```python
from build123d import *

# Parameters (mm, degrees)
SKETCH1_R           = 1.7
SKETCH1_W           = 5.3
SKETCH1_H           = 7.2
BOSS_EXTRUDE2_DEPTH = 6
SKETCH1_4_W         = 5.3
SKETCH1_4_H         = 7.2
CUT_EXTRUDE1_DEPTH  = 3.8
FILLET2_R           = 4
FILLET3_R           = 2


with BuildPart() as part:
    # Sketch1 → Boss-Extrude2 (new body)
    # profile 1 of 2: a face of its own
    with BuildSketch(Plane(origin=(0, 0, 0), x_dir=(1, 0, 0), z_dir=(0, 1, 0))):
        Polygon((-25.7, 5), (-25.7, -5), (25.7, -5), (25.7, 5), (2.65, 5), (2.65, -2.2), (-2.65, -2.2), (-2.65, 5), align=None)
        with Locations(Location((-20, 0, 0), (0, 0, 270))):
            Circle(SKETCH1_R, mode=Mode.SUBTRACT)
        with Locations(Location((20, 0, 0), (0, 0, 270))):
            Circle(SKETCH1_R, mode=Mode.SUBTRACT)
    # profile 2 of 2: a face of its own
    with BuildSketch(Plane(origin=(0, 0, 0), x_dir=(1, 0, 0), z_dir=(0, 1, 0))):
        with Locations((0, 1.4)):
            Rectangle(SKETCH1_W, SKETCH1_H)
    extrude(amount=BOSS_EXTRUDE2_DEPTH)

    # Sketch1_4 → Cut-Extrude1 (cut)
    with BuildSketch(Plane(origin=(0, 0, 0), x_dir=(1, 0, 0), z_dir=(0, 1, 0))):
        with Locations((0, 1.4)):
            Rectangle(SKETCH1_4_W, SKETCH1_4_H)
    extrude(amount=CUT_EXTRUDE1_DEPTH, mode=Mode.SUBTRACT)

    # Fillet2
    fillet2_edges = [part.edges().sort_by_distance(p)[0] for p in [
        (-25.7, 3, -5),
        (25.7, 3, -5),
    ]]
    fillet(fillet2_edges, radius=FILLET2_R)

    # Fillet3
    fillet3_edges = [part.edges().sort_by_distance(p)[0] for p in [
        (25.7, 3, 5),
        (-25.7, 3, 5),
    ]]
    fillet(fillet3_edges, radius=FILLET3_R)


solid = part.part
```
Here's how the part is built. I have some questions about the finished solid (model axes, mm). A direction names the side the tool comes from. Give positions to 0.01 mm unless a question says otherwise; leave off trailing zeros. Order: outer loops, then holes, each group sorted by start corner. A loop starts at its lowest first (then second) coordinate and runs counter-clockwise, first axis right, second up. Notation, with made-up numbers: M 80.25,-27.5 L 126.25,-27.5 A13 cw 126.25,-2.5 Z; hole C -32,-34 d3. An arc over 180 degrees is marked long. Use a Markdown table: item, result. Add a question column.
1. Suppose I cut it at B-B (x = 20). List the corners of the cut face in (y, z) for me, and give its area (3 significant figures).
2. If we mould it in two halves opening along Z, with no side actions, what happens to faces 1 (the flat face through (0, 4, -5)), 2 (the cylindrical face through (21.686, 2.958, -0.221)), 3 (the flat face through (0, 0, 3))? For each: +Z half, -Z half, draft (parallel to the pull), parting line (faces both ways), or undercut.
3. On a 3-axis mill with a long thin cutter (end or side, diameter ignored), from which of +Z, -Z, +X, -X, +Y, -Y can I reach the whole of each face in a straight line? I mean faces 4 (the flat face through (-2.65, 2, -1)), 5 (the flat face through (-25.7, 3, 1)). Say none if no direction works.
4. Suppose I cut it at A-A (y = 5.45). List the corners of the cut face in (x, z) for me.
5. I need wall thicknesses on probe 1 along X at (y, z) = (2.35, 0); probe 2 along X at (y, z) = (4.5, 0); probe 3 along X at (y, z) = (1.1, -2). Which ranges of each line are inside material? Lowest first, please. Write a range as from..to.
6. Suppose I cut it at C-C (z = -3.5). List the corners of the cut face in (x, y) for me, and give its area (3 significant figures).
7. For pin 1 Ø5.5 at (x, z) = (-20, 0) entering from +Y; pin 2 Ø2.5 at (x, z) = (-1, -2.5) entering from -Y; pin 3 Ø1 at (x, y) = (2, 2.5) entering from -Z, each with a flat end and sliding along its axis, tell me the tip position at first contact or that it passes through.
8. Suppose I cut it at D-D (y = 1). List the corners of the cut face in (x, z) for me.
Results list:
| question | item | result |
|---|---|---|
| 1 | outline | M 0,-5 L 6,-5 L 6,-1.7 L 0,-1.7 Z; M 0,1.7 L 6,1.7 L 6,5 L 0,5 Z |
| 1 | area | 39.6 mm² |
| 2 | face 1 | -Z half |
| 2 | face 2 | undercut |
| 2 | face 3 | draft |
| 3 | face 4 | -Z, -Y |
| 3 | face 5 | +Z, -Z, -X, +Y, -Y |
| 4 | outline | M -25.7,-1 A4 ccw -21.7,-5 L 21.7,-5 A4 ccw 25.7,-1 L 25.7,3 A2 ccw 23.7,5 L -23.7,5 A2 ccw -25.7,3 Z; hole C -20,0 d3.4; hole C 20,0 d3.4 |
| 5 | probe 1 | x = -25.7..-21.7, -18.3..-2.65, 2.65..18.3, 21.7..25.7 |
| 5 | probe 2 | x = -25.7..-21.7, -18.3..18.3, 21.7..25.7 |
| 5 | probe 3 | x = -25.57..-2.65, 2.65..25.57 |
| 6 | outline | M -24.82,0 L -2.65,0 L -2.65,3.8 L 2.65,3.8 L 2.65,0 L 24.82,0 L 24.82,6 L -24.82,6 Z |
| 6 | area | 278 mm² |
| 7 | pin 1 | stops at y = 6 |
| 7 | pin 2 | stops at y = 3.8 |
| 7 | pin 3 | stops at z = 2.2 |
| 8 | outline | M -25.7,-1 A4 ccw -21.7,-5 L -2.65,-5 L -2.65,2.2 L 2.65,2.2 L 2.65,-5 L 21.7,-5 A4 ccw 25.7,-1 L 25.7,3 A2 ccw 23.7,5 L -23.7,5 A2 ccw -25.7,3 Z; hole C -20,0 d3.4; hole C 20,0 d3.4 |
